from build123d import *

# Parameters (mm, degrees)
F0_R     = 1.524
F0_R_2   = 1.778
F0_R_3   = 6.35
F1_DEPTH = 5.842


with BuildPart() as f1:
    # F0 (on Top) → F1 (new body)
    with BuildSketch(Plane.XY):
        with BuildLine():
            Line((16.51, 19.05), (-16.51, 19.05))
            ThreePointArc((-16.51, 19.05), (-18.306051, 18.306051), (-19.05, 16.51))
            Line((-19.05, 16.51), (-19.05, -16.51))
            ThreePointArc((-19.05, -16.51), (-18.306051, -18.306051), (-16.51, -19.05))
            Line((-16.51, -19.05), (16.51, -19.05))
            ThreePointArc((16.51, -19.05), (18.306051, -18.306051), (19.05, -16.51))
            Line((19.05, -16.51), (19.05, 16.51))
            ThreePointArc((19.05, 16.51), (18.306051, 18.306051), (16.51, 19.05))
        make_face()
        with Locations((-12, -12)):
            Circle(F0_R, mode=Mode.SUBTRACT)
        with Locations((0, -9.779)):
            Circle(F0_R_2, mode=Mode.SUBTRACT)
        with Locations((12, -12)):
            Circle(F0_R, mode=Mode.SUBTRACT)
        with Locations((-9.779, 0)):
            Circle(F0_R_2, mode=Mode.SUBTRACT)
        with Locations((-12, 12)):
            Circle(F0_R, mode=Mode.SUBTRACT)
        Circle(F0_R_3, mode=Mode.SUBTRACT)
        with Locations((9.779, 0)):
            Circle(F0_R_2, mode=Mode.SUBTRACT)
        with Locations((0, 9.779)):
            Circle(F0_R_2, mode=Mode.SUBTRACT)
        with Locations((12, 12)):
            Circle(F0_R, mode=Mode.SUBTRACT)
    extrude(amount=F1_DEPTH)


solid = f1.part
Work out the finished part from the listing and answer in its coordinate system (mm). Round coordinates to 2 decimals unless told otherwise and drop trailing zeros. Write each loop counter-clockwise with the first axis right and the second up, starting at its lowest first coordinate (ties: lowest second). Pieces come first, ordered by that corner, then holes. Notation, with made-up numbers: (-19.5, 50.25) - (35.5, 50.25) arc R34 ccw to (35.5, 82.25) - close; hole circle Ø9 at (86.25, 40.5). An arc over 180 degrees is marked (long way). Answer in a Markdown table with one row per item. Add a question column.
1. A cutting plane is placed at C-C, the plane x = 0. Determine the outline of the cut face in (y, z), and give its area (3 significant figures).
2. The mould has two halves that part along X. Classify faces 1 (the cylindrical face through (-11.19, -1.08, 2.88)), 2 (the cylindrical face through (-18.286, 18.326, 2.88)), 3 (the flat face through (-5, 5, 0)): +X half, -X half, draft (parallel to the pull), parting line (faces both ways), or undercut.
3. Find the intervals of material crossed by line 1 along Y through (x, z) = (0, 2); line 2 along Y through (x, z) = (-12, 1.6); line 3 along X through (y, z) = (12.5, 4.25), in increasing order. Write a range as from..to.
4. A cutting plane is placed at A-A, the plane x = 12. Determine the outline of the cut face in (y, z), and give its area (3 significant figures).
Worked out:
| question | item | result |
|---|---|---|
| 1 | outline | (-19.05, 0) - (-11.56, 0) - (-11.56, 5.84) - (-19.05, 5.84) - close; (-8, 0) - (-6.35, 0) - (-6.35, 5.84) - (-8, 5.84) - close; (6.35, 0) - (8, 0) - (8, 5.84) - (6.35, 5.84) - close; (11.56, 0) - (19.05, 0) - (19.05, 5.84) - (11.56, 5.84) - close |
| 1 | area | 107 mm^2 |
| 2 | face 1 | undercut |
| 2 | face 2 | -X half |
| 2 | face 3 | draft |
| 3 | line 1 | -19.05..-11.56, -8..-6.35, 6.35..8, 11.56..19.05 |
| 3 | line 2 | -19.05..-13.52, -10.48..10.48, 13.52..19.05 |
| 3 | line 3 | -19.05..-13.44, -10.56..10.56, 13.44..19.05 |
| 4 | outline | (-19.05, 0) - (-13.52, 0) - (-13.52, 5.84) - (-19.05, 5.84) - close; (-10.48, 0) - (10.48, 0) - (10.48, 5.84) - (-10.48, 5.84) - close; (13.52, 0) - (19.05, 0) - (19.05, 5.84) - (13.52, 5.84) - close |
| 4 | area | 187 mm^2 |
